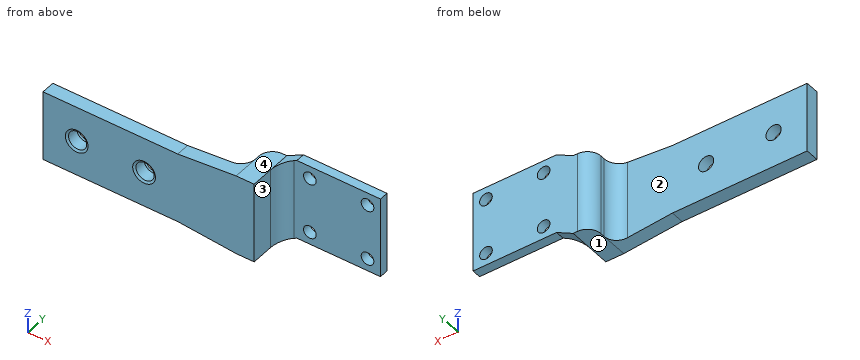
from build123d import *

# Parameters (mm, degrees)
BODY_DEPTH                           = 38.1
F_13_64_0_20313_DIAMETER_HOLE1_D     = 5.159502
F_13_64_0_20313_DIAMETER_HOLE1_DEPTH = 3.556
F_13_64_0_20313_DIAMETER_HOLE1_TIP   = 1.550070783
CHAMFER1_SIZE                        = 0.635
CHAMFER1_SIZE2                       = 0.366617421
REACHER_DEPTH                        = 3.81
SKETCH13_W                           = 5.08
SKETCH13_H                           = 22.987
BOSS_EXTRUDE4_DEPTH                  = 8.89
SKETCH11_R                           = 1.7907
BOSS_EXTRUDE3_DEPTH                  = 2.54
FILLET1_R                            = 3.81


with BuildPart() as part:
    # Profile → Body (new body)
    with BuildSketch(Plane(origin=(0, 0, 0), x_dir=(0, 0, -1), z_dir=(1, 0, 0))):
        Polygon((20, -1.905), (20, 1.905), (0, 1.905), (0, -1.905), (4.92, -1.905), (10, -1.905), (15.08, -1.905), align=None)
    extrude(amount=BODY_DEPTH)

    # 13/64 (0.20313) Diameter Hole1
    with Locations(Plane(origin=(0, -1.905, 0), x_dir=(-1, 0, 0), z_dir=(0, -1, 0))):
        with Locations((-28.575, 10), (-9.525, 10)):
            Hole(F_13_64_0_20313_DIAMETER_HOLE1_D / 2, depth=F_13_64_0_20313_DIAMETER_HOLE1_DEPTH)
            with Locations((0, 0, -(F_13_64_0_20313_DIAMETER_HOLE1_DEPTH + F_13_64_0_20313_DIAMETER_HOLE1_TIP / 2))):  # 118° drill point
                Cone(0, F_13_64_0_20313_DIAMETER_HOLE1_D / 2, F_13_64_0_20313_DIAMETER_HOLE1_TIP, mode=Mode.SUBTRACT)

    # Chamfer1
    chamfer1_edges = [part.edges().sort_by_distance(p)[0] for p in [
        (6.945249, -1.905, -10),
        (25.995249, -1.905, -10),
    ]]
    chamfer1_side = [part.faces().sort_by_distance(p)[0] for p in [
        (19.05, -1.905, -10),
    ]]
    chamfer(chamfer1_edges, length=CHAMFER1_SIZE, length2=CHAMFER1_SIZE2, reference=chamfer1_side[0])

    # Sketch9 → Reacher (add)
    with BuildSketch(Plane(origin=(0, -1.905, 0), x_dir=(1, 0, 0), z_dir=(0, 1, 0))):
        Polygon((54.61, 21.4935), (38.1, 20), (38.1, 0), (54.61, -1.4935), (59.69, -1.4935), (59.69, 21.4935), align=None)
    extrude(amount=REACHER_DEPTH)

    # Sketch13 → Boss-Extrude4 (add)
    with BuildSketch(Plane(origin=(0, 1.905, 0), x_dir=(1, 0, 0), z_dir=(0, 1, 0))):
        with Locations((57.15, 10)):
            Rectangle(SKETCH13_W, SKETCH13_H)
    extrude(amount=BOSS_EXTRUDE4_DEPTH)

    # Sketch11 → Boss-Extrude3 (add)
    with BuildSketch(Plane(origin=(0, 10.795, 0), x_dir=(1, 0, 0), z_dir=(0, 1, 0))):
        Polygon((64.389, -4.0335), (88.011, -4.0335), (88.011, 18.9535), (64.389, 18.9535), (59.69, 21.4935), (59.69, -1.4935), align=None)
        with Locations((68.056282873, 15.3848)):
            Circle(SKETCH11_R, mode=Mode.SUBTRACT)
        with Locations((84.343717127, 15.3848)):
            Circle(SKETCH11_R, mode=Mode.SUBTRACT)
        with Locations((84.343717127, -0.4648)):
            Circle(SKETCH11_R, mode=Mode.SUBTRACT)
        with Locations((68.056282873, -0.4648)):
            Circle(SKETCH11_R, mode=Mode.SUBTRACT)
    extrude(amount=-BOSS_EXTRUDE3_DEPTH)

    # Fillet1
    fillet1_edges = [part.edges().sort_by_distance(p)[0] for p in [
        (54.61, 1.905, -10),
        (54.61, 10.795, -10),
        (59.69, 8.255, -10),
    ]]
    fillet(fillet1_edges, radius=FILLET1_R)


solid = part.part
The listing builds one solid part. Answer for the finished solid, in the listing's coordinates (mm). Face numbers are marked on the shaded views. A direction names the side the tool comes from. Give positions to 0.01 mm unless a question says otherwise; leave off trailing zeros. Loops run counter-clockwise (first coordinate to the right, second up) from the corner with the lowest first, then second, coordinate; pieces in that order, holes last. Notation, with made-up numbers: M 6.5,-33 L 39.5,-33 A13 ccw 39.5,-14 Z; hole C 50.5,-32.5 d9. An arc over 180 degrees is marked long. Answer as CSV lines item,"result".
Item 1: The part is cut by section B-B (z = -10). Give the vertices of the cut face in (x, y) (3 decimals), and give its area (3 significant figures).
Values follow:
outline,"M 0,-1.905 L 6.31,-1.905 L 6.945,-1.538 L 6.945,1.651 L 7.368,1.905 L 0,1.905 Z; M 11.682,1.905 L 12.105,1.651 L 12.105,-1.538 L 12.74,-1.905 L 25.36,-1.905 L 25.995,-1.538 L 25.995,1.651 L 26.418,1.905 Z; M 30.732,1.905 L 31.155,1.651 L 31.155,-1.538 L 31.79,-1.905 L 59.69,-1.905 L 59.69,4.445 A3.81 cw 63.5,8.255 L 88.011,8.255 L 88.011,10.795 L 58.42,10.795 A3.81 ccw 54.61,6.985 L 54.61,5.715 A3.81 cw 50.8,1.905 Z"
area,"308 mm^2"
Item 2: The part is cut by section C-C (y = 9.5). Give the vertices of the cut face in (x, z), and give its area (3 significant figures).
Values follow:
outline,"M 55.56,-21.49 L 59.69,-21.49 L 64.39,-18.95 L 88.01,-18.95 L 88.01,4.03 L 64.39,4.03 L 59.69,1.49 L 55.56,1.49 Z; hole C 68.06,-15.38 d3.58; hole C 68.06,0.46 d3.58; hole C 84.34,-15.38 d3.58; hole C 84.34,0.46 d3.58"
area,"706 mm^2"
Item 3: Straight lines are drawn through the part: line 1 along X through (y, z) = (0.5, -10); line 2 along Y through (x, z) = (65, -12.5) (3 decimals); line 3 along Z through (x, y) = (57, 0.75). For each, find the intervals that lie inside material, in ascending order. Write a range as [from, to].
Values follow:
line 1,"x = [0, 6.95], [12.1, 26], [31.15, 59.69]"
line 2,"y = [8.255, 10.795]"
line 3,"z = [-21.49, 1.49]"
Item 4: Which of the six approach directions +Z, -Z, +X, -X, +Y, -Y give full straight-line access (tool end or side, diameter ignored) to the marked faces 1, 2, 3 and 4?
Values follow:
face 1,"-Z, +X, -X, +Y, -Y"
face 2,"+Z, -Z, -X, +Y"
face 3,"+Z, -Z, +X, -Y"
face 4,"+Z, -X, +Y, -Y"
Item 5: The part is cut by section A-A (z = -5.5). Give the vertices of the cut face in (x, y) (3 decimals).
Values follow:
outline,"M 0,-1.905 L 59.69,-1.905 L 59.69,4.445 A3.81 cw 63.5,8.255 L 88.011,8.255 L 88.011,10.795 L 58.42,10.795 A3.81 ccw 54.61,6.985 L 54.61,5.715 A3.81 cw 50.8,1.905 L 0,1.905 Z"
Item 6: The part is cut by section D-D (y = 3.5). Give the vertices of the cut face in (x, z), and give its area (3 significant figures).
Values follow:
outline,"M 53.9,-21.43 L 54.61,-21.49 L 59.69,-21.49 L 59.69,1.49 L 54.61,1.49 L 53.9,1.43 Z"
area,"133 mm^2"
Item 7: Given pin 1 Ø4.5 at (x, z) = (84.34, -15.38) entering from -Y (3 decimals); pin 2 Ø3 at (x, y) = (79.5, 9.5) entering from -Z; pin 3 Ø2.5 at (x, y) = (57, 3.5) entering from +Z; pin 4 Ø6 at (x, y) = (28, 7.5) entering from -Z, each flat-ended and moving along its own axis, determine where each tip first touches the part or whether it passes through.
Values follow:
pin 1,"stops at y = 8.255"
pin 2,"stops at z = -18.95"
pin 3,"stops at z = 1.49"
pin 4,"passes through"
